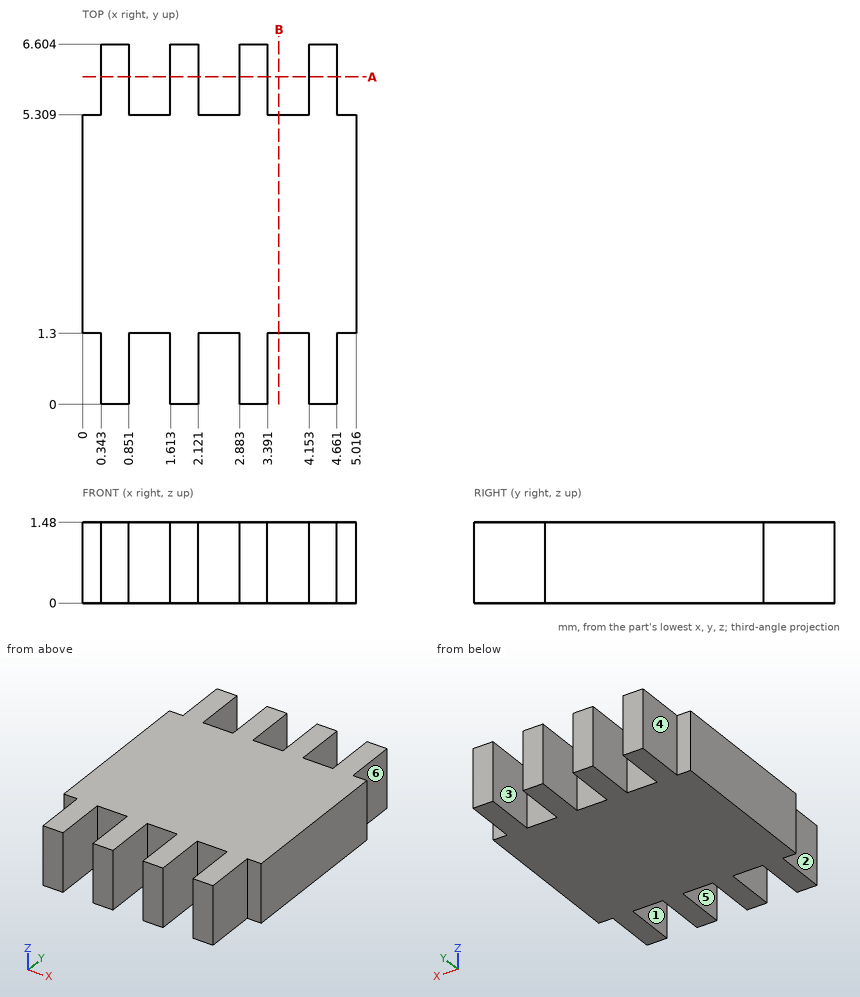
The figure shows three views and two pictorial views of one solid part (mm, origin at its lowest corner). Answer the questions. A direction names the side the tool comes from. Give positions to 0.01 mm unless a question says otherwise; leave off trailing zeros. Write each loop counter-clockwise with the first axis right and the second up, starting at its lowest first coordinate (ties: lowest second). Pieces come first, ordered by that corner, then holes. Notation, with made-up numbers: (56, 82.25) - (91, 82.25) arc R28 cw to (91, 110.25) - close; hole circle Ø9 at (-35, -30.5). An arc over 180 degrees is marked (long way). Use CSV: the item, a comma, the result in double quotes. Start each with the question number.
Item 1: For the marked faces 1, 2 and 3, determine the directions among +Z, -Z, +X, -X, +Y, -Y from which every point of the face is accessible in a straight line to the end or side of a thin tool.
Item 2: The mould has two halves that part along X. Classify the marked faces 4, 5 and 6: pulls with the +X half, pulls with the -X half, needs draft (parallel to the pull), parting line crosses it, or undercut.
Item 3: The part is cut by section B-B, the plane x = 3.6. Give the vertices of the cut face in (y, z).
Item 4: Flat-ended cylindrical pins translate along their axes: P1, Ø0.6, axis at x = 1, z = 1, coming from the -Y side; P2, Ø0.6, axis at y = 6, z = 0.5, coming from the -X side. Find the tip coordinate at first contact, or state that the pin passes through.
Item 5: The part is cut by section A-A, the plane y = 6. Give the vertices of the cut face in (x, z).
Item 6: Consider line 1 (X direction, y = 5.75, z = 0.6); line 2 (Y direction, x = 0.9, z = 0.65). Determine where each line is inside the solid, lowest interval first.
Taken from the geometry:
1,face 1,"+Z, -Z, -Y"
1,face 2,"+Z, -Z, -X, -Y"
1,face 3,"+Z, -Z, +Y"
2,face 4,"pulls with the -X half"
2,face 5,"undercut"
2,face 6,"pulls with the +X half"
3,outline,"(1.3, 0) - (5.31, 0) - (5.31, 1.48) - (1.3, 1.48) - close"
4,P1,"y = 0"
4,P2,"x = 0.34"
5,outline,"(0.34, 0) - (0.85, 0) - (0.85, 1.48) - (0.34, 1.48) - close; (1.61, 0) - (2.12, 0) - (2.12, 1.48) - (1.61, 1.48) - close; (2.88, 0) - (3.39, 0) - (3.39, 1.48) - (2.88, 1.48) - close; (4.15, 0) - (4.66, 0) - (4.66, 1.48) - (4.15, 1.48) - close"
6,line 1,"0.34 to 0.85, 1.61 to 2.12, 2.88 to 3.39, 4.15 to 4.66"
6,line 2,"1.3 to 5.31"
